Autodesk Inventor part; units mm, degrees
ref_plane "Work Plane1" through (-30, 0, -30) normal (0, 1, 0) x (0, 0, 1)
ref_plane "YZ Plane" through (0, 0, 0) normal (1, 0, 0) x (0, 1, 0)
ref_plane "XZ Plane" through (0, 0, 0) normal (0, 1, 0) x (-1, 0, 0)
sketch "Sketch1" plane through (0, 0, 0) normal (0, 1, 0) x (-1, 0, 0)
  line L0 (-30, -30) -> (30, -30)
  line L1 (30, -30) -> (30, 30)
  line L2 (30, 30) -> (-30, 30)
  line L3 (-30, 30) -> (-30, -30)
  line L4 (-30, -30) -> (30, 30) construction
  line L5 (30, -30) -> (-30, 30) construction
  circle A0 centre (0, 0) radius 7.5
  dimension "d0" = 60
  dimension "d1" = 60
  dimension "d13" = 15
extrude "Extrusion1" add sketch "Sketch1" along normal blind 12 contours L3 L2 L1 L0 | A0
sketch "Sketch2" plane through (0, 12, 0) normal (0, 1, 0) x (1, 0, 0)
  line L0 (30, 30) -> (-30, 30)
  line L1 (-30, 30) -> (-30, -30)
  line L2 (-30, -30) -> (30, -30)
  line L3 (30, -30) -> (30, 30)
  line L4 (25, -25) -> (-25, -25)
  line L5 (-25, -25) -> (-25, 25)
  line L6 (-25, 25) -> (25, 25)
  line L7 (25, 25) -> (25, -25)
  line L8 (25, -25) -> (-25, 25) construction
  line L9 (-25, -25) -> (25, 25) construction
  line L10 (0, -25) -> (0, 25)
  line L11 (-25, 0) -> (25, 0)
  point P0 (0, 0)
  point P1 (0, 0)
  dimension "d4" = 50
  dimension "d5" = 50
hole "Hole1" at (-25, 12, 25) at (-25, 12, -25) at (25, 12, -25) at (25, 12, 25) at (0, 12, 25) at (0, 12, 0) at (-25, 12, 0) at (0, 12, -25) at (25, 12, 0) direction (0, -1, 0) diameter 2.9 depth 10 tip angle 118
chamfer "Chamfer1" distance 2 angle 45 4 edges at (30, 6, 30) (30, 6, -30) (-30, 6, -30) (-30, 6, 30)
sketch "Sketch3" plane through (0, 12, 0) normal (0, 1, 0) x (1, 0, 0)
  line L0 (-28, -30) -> (-30, -28)
  line L1 (-28, -30) -> (28, -30)
  line L2 (30, -28) -> (28, -30)
  line L3 (30, -28) -> (30, 28)
  line L4 (28, 30) -> (30, 28)
  line L5 (28, 30) -> (-28, 30)
  line L6 (-30, 28) -> (-28, 30)
  line L7 (-30, 28) -> (-30, -28)
  circle A0 centre (0, 25) radius 1.45
  circle A1 centre (0, 0) radius 1.45
  circle A2 centre (25, -25) radius 1.45
  circle A3 centre (-25, 25) radius 1.45
  circle A4 centre (-25, -25) radius 1.45
  circle A5 centre (25, 25) radius 1.45
  circle A6 centre (0, -25) radius 1.45
  circle A7 centre (-25, 0) radius 1.45
  circle A8 centre (25, 0) radius 1.45
  line L8 (-30, 28) -> (-30, -28)
  line L9 (-30, -24.5) -> (-45, -24.5)
  line L10 (-45, -24.5) -> (-45, -6.5)
  line L11 (-45, -6.5) -> (-30, -6.5)
  line L12 (-30, -6.5) -> (-30, -24.5)
  line L13 (-30, 7) -> (-45, 7)
  line L14 (-45, 7) -> (-45, 22)
  line L15 (-45, 22) -> (-30, 22)
  line L16 (-30, 22) -> (-30, 7)
  line L17 (-45, 7) -> (-49, 7)
  line L18 (-49, 7) -> (-49, 22)
  line L19 (-49, 22) -> (-45, 22)
  line L20 (-45, 22) -> (-45, 7)
  dimension "d17" = 15
  dimension "d18" = 18
  dimension "d19" = 5.5
  dimension "d20" = 15
  dimension "d21" = 8
  dimension "d22" = 19
ref_plane "Work Plane1" through (-30, 0, -30) normal (0, 1, 0) x (0, 0, 1)
extrude "Extrusion2" add sketch "Sketch3" against normal up to surface (12 mm away) contours L9 L10 L11 L7 | L13 L14 L15 L7 | L17 L18 L19 L14
sketch "Sketch4" plane through (-30, 12, -22) normal (0, 0, -1) x (-1, 0, 0)
  line L0 (15, 0) -> (15, -12)
  line L1 (19, -12) -> (0, -12)
  line L2 (19, 0) -> (19, -12)
  line L3 (0, 0) -> (19, 0)
  line L4 (0, -12) -> (0, 0)
  circle A0 centre (9.5, -6) radius 3.2291
  point P0 (-30, -12)
extrude "Extrusion3" cut sketch "Sketch4" against normal through all contours A0
properties part number "00_XY_stage-CHUO_SEIKI_LD-647-R1-Top"
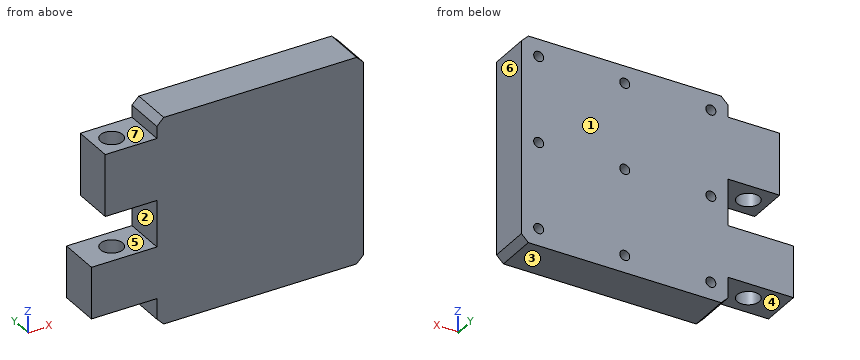
CAD build for the part. Positions are in the model's coordinates, mm. Face numbers are marked on the shaded views. A direction names the side the tool comes from. Round coordinates to 2 decimals unless told otherwise and drop trailing zeros. Write each loop counter-clockwise with the first axis right and the second up, starting at its lowest first coordinate (ties: lowest second). Pieces come first, ordered by that corner, then holes. Notation, with made-up numbers: M -7.75,-9 L 35.25,-9 A13 cw 35.25,-3 Z; hole C -19,81.25 d1. An arc over 180 degrees is marked long. Put each result on its own line as item: value. Start each with the question number.
1) Saw through at C-C, the plane z = 21. Write the cut outline in (x, y), and give its area (3 significant figures).
2) 3-axis set-ups, long thin cutter, end or side, ignore diameter. For the marked faces 4, 5, 6 and 7: which of +Z, -Z, +X, -X, +Y, -Y reach the whole face in a straight line?
3) Drill centre lines: probe 1 along X at (y, z) = (9.75, 25); probe 2 along Z at (x, y) = (-43.5, 3.5). Where is each one in solid material? Low to high. Write a range as [from, to].
4) Saw through at A-A, the plane y = 6. Count the separate pieces of the cut face and the enclosed holes in it, and give its area (3 significant figures).
5) Saw through at D-D, the plane z = -6. Write the cut outline in (x, y).
6) Pin check, flat tips, straight feed: pin 1 Ø4 at (x, y) = (-37.5, 11) entering from +Z; pin 2 Ø5 at (y, z) = (5.5, 9.5) entering from -X; pin 3 Ø1 at (y, z) = (9, 26.5) entering from -X. Stop position of each tip, or through.
7) Pull direction Z, two halves, no side cores. Call the marked faces 1, 2 and 3: pulls with the +Z half, pulls with the -Z half, needs draft (parallel to the pull), parting line crosses it, or undercut.
8) Saw through at B-B, the plane x = -39.5. Write the cut outline in (y, z), and give its area (3 significant figures).
Resolved:
1. outline: M -45,0 L 30,0 L 30,12 L -45,12 Z; hole C -39.5,6 d6.46
1. area: 867 mm²
2. face 4: -Z, -X, +Y, -Y
2. face 5: -X, +Y, -Y
2. face 6: +Z, -Z, +X, +Y, -Y
2. face 7: +Z, -X, +Y, -Y
3. probe 1: [-30, -26.45], [-23.55, -1.45], [1.45, 23.55], [26.45, 30]
3. probe 2: [-22, -7], [6.5, 24.5]
4. separate pieces: 3
4. enclosed holes: 9
4. area: 3,870 mm²
5. outline: M -30,0 L 30,0 L 30,12 L -30,12 Z
6. pin 1: z = 24.5
6. pin 2: x = -45
6. pin 3: x = -30
7. face 1: needs draft
7. face 2: undercut
7. face 3: pulls with the -Z half
8. outline: M 0,-22 L 2.77,-22 L 2.77,-7 L 0,-7 Z; M 0,6.5 L 2.77,6.5 L 2.77,24.5 L 0,24.5 Z; M 9.23,-22 L 12,-22 L 12,-7 L 9.23,-7 Z; M 9.23,6.5 L 12,6.5 L 12,24.5 L 9.23,24.5 Z
8. area: 183 mm²
